Read the model definition and answer for the solid it produces. Units are mm, in the model's axes. Round coordinates to 2 decimals unless told otherwise and drop trailing zeros. Order: outer loops, then holes, each group sorted by start corner. A loop starts at its lowest first (then second) coordinate and runs counter-clockwise, first axis right, second up. Notation, with made-up numbers: (10, 40) - (39, 40) arc R4 ccw to (39, 46) - close; hole circle Ø5 at (28.25, 56). An arc over 180 degrees is marked (long way). Answer as a JSON object with one key per item and string values. Group by question number.
Q1. A cutting plane is placed at C-C on y = 5.5. Determine the outline of the cut face in (x, z).
Q2. Consider line 1 (X direction, y = 14.5, z = 0.1); line 2 (Z direction, x = -0.55, y = 24). Determine where each line is inside the solid, lowest interval first.
Q3. A cutting plane is placed at B-B on z = -0.6. Determine the outline of the cut face in (x, y).
Q4. A cutting plane is placed at A-A on x = 0.6. Determine the outline of the cut face in (y, z), and give its area (3 significant figures).
Autodesk Inventor part; units mm, degrees
ref_plane "YZ Plane" through (0, 0, 0) normal (1, 0, 0) x (0, 1, 0)
ref_plane "XZ Plane" through (0, 0, 0) normal (0, 1, 0) x (-1, 0, 0)
ref_plane "XY Plane" through (0, 0, 0) normal (0, 0, 1) x (1, 0, 0)
sketch "Sketch1" plane through (0, 0, 0) normal (0, 1, 0) x (-1, 0, 0)
  circle A0 centre (0, 0) radius 1
  dimension "d0" = 2
extrude "Extrusion1" add sketch "Sketch1" along normal blind 26
ref_plane "Work Plane1" through (0, -30, 0) normal (0, -1, 0) x (1, 0, 0)
move faces "Move1" translate (0, -0.25, 0) faces at (-0.5848, 0, -0.397)
move faces "Move2" translate (0, -0.93, 0) faces at (-0.2495, 26, 0.221)
properties part number "LOOP2_COLL"
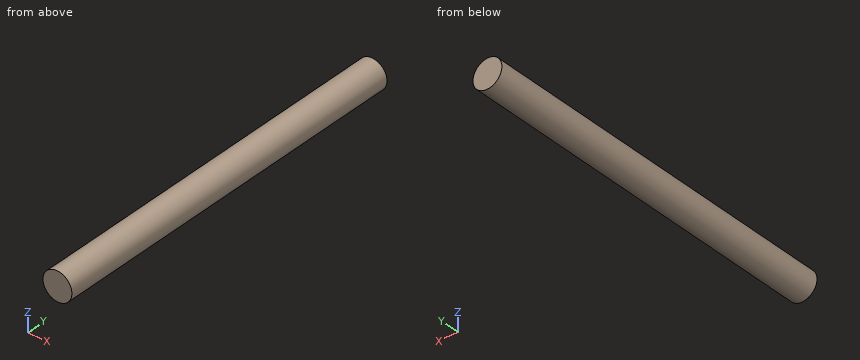
Result set:
{
 "1": {"outline": "circle Ø2 at (0, 0)"},
 "2": {"line 1": "x = -0.99 to 0.99", "line 2": "z = -0.84 to 0.84"},
 "3": {"outline": "(-0.8, -0.25) - (0.8, -0.25) - (0.8, 25.07) - (-0.8, 25.07) - close"},
 "4": {"outline": "(-0.25, -0.8) - (25.07, -0.8) - (25.07, 0.8) - (-0.25, 0.8) - close", "area": "40.5 mm²"}
}
